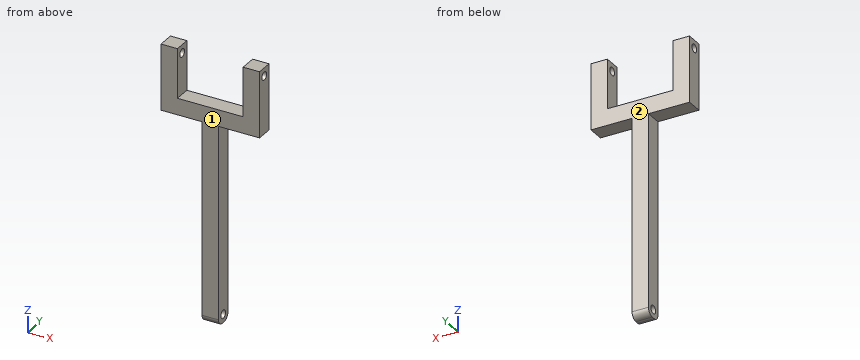
```python
from build123d import *

# Parameters (mm, degrees)
SKETCH1_W                = 12.7
SKETCH1_H                = 12.7
BOSS_EXTRUDE1_DEPTH      = 86.36
BOSS_EXTRUDE1_DEPTH_BACK = 80.01
SKETCH4_W                = 12.7
SKETCH4_H                = 12.7
BOSS_EXTRUDE2_DEPTH      = 38.1
SKETCH5_W                = 12.7
SKETCH5_H                = 12.7
BOSS_EXTRUDE3_DEPTH      = 50.8
SKETCH6_R                = 3.175
CUT_EXTRUDE1_DEPTH       = 16.51
SKETCH7_R                = 3.175
CUT_EXTRUDE2_DEPTH       = 45.45
FILLET1_R                = 5.08


with BuildPart() as part:
    # Sketch1 → Boss-Extrude1 (new body, two sides)
    with BuildSketch(Plane.XY) as boss_extrude1_sk:
        Rectangle(SKETCH1_W, SKETCH1_H)
    extrude(amount=BOSS_EXTRUDE1_DEPTH)
    extrude(boss_extrude1_sk.sketch, amount=-BOSS_EXTRUDE1_DEPTH_BACK)

    # Sketch4 → Boss-Extrude2 (add, symmetric)
    with BuildSketch(Plane(origin=(0, 0, 0), x_dir=(0, 0, -1), z_dir=(1, 0, 0))):
        with Locations((-80.01, 0)):
            Rectangle(SKETCH4_W, SKETCH4_H)
    extrude(amount=BOSS_EXTRUDE2_DEPTH, both=True)

    # Sketch5 → Boss-Extrude3 (add)
    with BuildSketch(Plane(origin=(0, 0, 73.66), x_dir=(-1, 0, 0), z_dir=(0, 0, -1))):
        with Locations((-31.75, 0)):
            Rectangle(SKETCH5_W, SKETCH5_H)
    boss_extrude3 = extrude(amount=-BOSS_EXTRUDE3_DEPTH)

    # Sketch6 → Cut-Extrude1 (cut)
    with BuildSketch(Plane.ZY.offset(-25.4)):
        with Locations((118.11, 0)):
            Circle(SKETCH6_R)
    cut_extrude1 = extrude(amount=-CUT_EXTRUDE1_DEPTH, mode=Mode.SUBTRACT)

    # Mirror1: Boss-Extrude3, Cut-Extrude1 across plane
    add(boss_extrude3.mirror(Plane(origin=(0, 0, 0), x_dir=(0, 0, 1), z_dir=(1, 0, 0))))
    add(cut_extrude1.mirror(Plane(origin=(0, 0, 0), x_dir=(0, 0, 1), z_dir=(1, 0, 0))), mode=Mode.SUBTRACT)

    # Sketch7 → Cut-Extrude2 (cut, through all)
    with BuildSketch(Plane.ZY.offset(6.35)):
        with Locations((-73.66, 0)):
            Circle(SKETCH7_R)
    extrude(amount=-CUT_EXTRUDE2_DEPTH, mode=Mode.SUBTRACT)

    # Fillet1
    fillet1_edges = [part.edges().sort_by_distance(p)[0] for p in [
        (0, 6.35, -80.01),
        (0, -6.35, -80.01),
    ]]
    fillet(fillet1_edges, radius=FILLET1_R)


solid = part.part
```
Source: CAD feature listing. Evaluate the final solid. Frame: model axes, mm. Face numbers are marked on the shaded views. Give positions to 0.01 mm unless a question says otherwise; leave off trailing zeros. Order: outer loops, then holes, each group sorted by start corner. A loop starts at its lowest first (then second) coordinate and runs counter-clockwise, first axis right, second up.
(1) Contact query for flat-ended pins moving along their axis: P1, Ø4, axis at x = -24.5, y = -1.5, coming from the -Z side; P2, Ø6, axis at y = -2.5, z = -27.5, coming from the +X side; P3, Ø8, axis at x = -9, z = 6, coming from the -Y side; P4, Ø4, axis at y = 1.5, z = 8, coming from the -X side. Output: stop coordinate, or through.
(2) Pull-direction query (Y, two-part tool) for the marked faces 1 and 2; classes: +Y half, -Y half, draft (parallel to the pull), parting line (faces both ways), or undercut.
(3) Section query D-D (z = -31.5). Return the cut outline in (x, y), plus the area to 3 significant figures.
(4) Section query B-B (x = 3). Return the cut outline in (y, z) (3 decimals), plus the area to 3 significant figures.
(5) Section query A-A (z = 110). Return the cut outline in (x, y), plus the area to 3 significant figures.
(6) Section query C-C (x = -22). Return the cut outline in (y, z), plus the area to 3 significant figures.
(7) Material intervals for line 1 along Y through (x, z) = (-35, 118.11) (3 decimals); line 2 along Z through (x, y) = (-31.5, 0) (3 decimals); line 3 along X through (y, z) = (-2.75, 99), sorted ascending.
Outcome:
1. P1: stops at z = 73.66
1. P2: stops at x = 6.35
1. P3: stops at y = -6.35
1. P4: stops at x = -6.35
2. face 1: -Y half
2. face 2: +Y half
3. outline: (-6.35, -6.35) - (6.35, -6.35) - (6.35, 6.35) - (-6.35, 6.35) - close
3. area: 161 mm2
4. outline: (-6.35, -74.93) arc R5.08 ccw to (-1.27, -80.01) - (1.27, -80.01) arc R5.08 ccw to (6.35, -74.93) - (6.35, 86.36) - (-6.35, 86.36) - close; hole circle Ø6.35 at (0, -73.66)
4. area: 2,070 mm2
5. outline: (-38.1, -6.35) - (-25.4, -6.35) - (-25.4, 6.35) - (-38.1, 6.35) - close; (25.4, -6.35) - (38.1, -6.35) - (38.1, 6.35) - (25.4, 6.35) - close
5. area: 323 mm2
6. outline: (-6.35, 73.66) - (6.35, 73.66) - (6.35, 86.36) - (-6.35, 86.36) - close
6. area: 161 mm2
7. line 1: y = -6.35 to -3.175, 3.175 to 6.35
7. line 2: z = 73.66 to 114.935, 121.285 to 124.46
7. line 3: x = -38.1 to -25.4, 25.4 to 38.1
